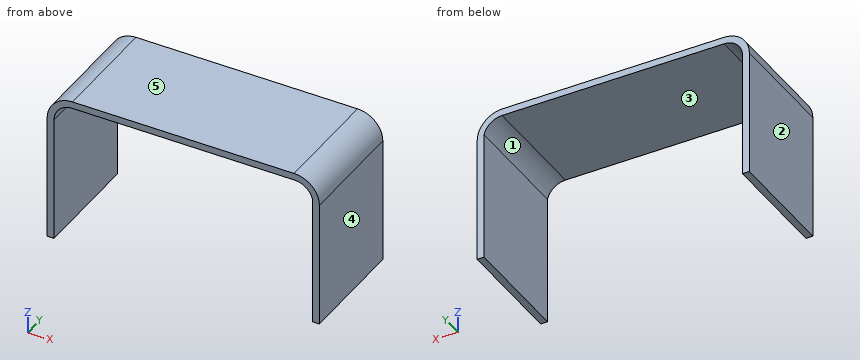
from build123d import *

# Parameters (mm, degrees)
F1_DEPTH = 147


with BuildPart() as f1:
    # F0 (on Front) → F1 (new body, symmetric)
    with BuildSketch(Plane.XZ):
        with BuildLine():
            Line((-1558.323113, 252.341221), (-1558.323113, -76.658779))
            Line((-1558.323113, -76.658779), (-1540.323113, -76.658779))
            Line((-1540.323113, -76.658779), (-1540.323113, 252.341221))
            ThreePointArc((-1540.323113, 252.341221), (-1526.264239, 286.282347), (-1492.323113, 300.341221))
            Line((-1492.323113, 300.341221), (-913.152471, 300.341221))
            ThreePointArc((-913.152471, 300.341221), (-883.16695, 289.822797), (-866.323113, 262.87741))
            Line((-866.323113, 262.87741), (-866.323113, -76.658779))
            Line((-866.323113, -76.658779), (-848.323113, -76.658779))
            Line((-848.323113, -76.658779), (-848.323113, 252.341221))
            ThreePointArc((-848.323113, 252.341221), (-867.654066, 299.010269), (-914.323113, 318.341221))
            Line((-914.323113, 318.341221), (-1492.323113, 318.341221))
            ThreePointArc((-1492.323113, 318.341221), (-1538.992161, 299.010269), (-1558.323113, 252.341221))
        make_face()
    extrude(amount=F1_DEPTH, both=True)


solid = f1.part
Verification items for the finished model (mm, model axes). Face numbers are marked on the shaded views. A direction names the side the tool comes from. Coordinates: 2 decimals unless noted, no trailing zeros. Loops run counter-clockwise (first coordinate to the right, second up) from the corner with the lowest first, then second, coordinate; pieces in that order, holes last. Notation, with made-up numbers: (-3, 63.25) -> (10, 63.25) arc R31 cw to (10, 99.25) -> close; hole circle Ø10 at (10, 56). An arc over 180 degrees is marked (long way). Answer as a JSON object with one key per item and string values. Group by question number.
Item 1: Sectioned sample at B-B on y = -24.5. Record the boundary of the cut face in (x, z), plus the area to 3 significant figures.
Item 2: Depth check by flat-ended pin: pin 1 (6 mm diameter, centred on x = -984, y = -61, fed in from -Z). Enter the tip coordinate at first touch or a pass-through.
Item 3: Sectioned sample at A-A on z = 241.5. Record the boundary of the cut face in (x, y), plus the area to 3 significant figures.
Item 4: Scan lines: probe 1 along X at (y, z) = (-63, 116.5); probe 2 along Z at (x, y) = (-996.5, -118); probe 3 along X at (y, z) = (-30, 274.5). Record each from-to range of solid material in increasing order.
Item 5: Tool access check on the marked faces 1 and 2. Record the directions out of +Z, -Z, +X, -X, +Y, -Y that give a thin tool (end or side, any length) a straight path to the whole face; none if there is none.
Item 6: Sectioned sample at C-C on x = -1265. Record the boundary of the cut face in (y, z).
Item 7: Mould release check, pull along X, two halves, no side actions. Record for the marked faces 3, 4 and 5: +X half, -X half, draft (parallel to the pull), parting line (faces both ways), or undercut.
Evaluation:
{
 "1": {"outline": "(-1558.32, -76.66) -> (-1540.32, -76.66) -> (-1540.32, 252.34) arc R48 cw to (-1492.32, 300.34) -> (-913.15, 300.34) arc R48 cw to (-866.32, 262.88) -> (-866.32, -76.66) -> (-848.32, -76.66) -> (-848.32, 252.34) arc R66 ccw to (-914.32, 318.34) -> (-1492.32, 318.34) arc R66 ccw to (-1558.32, 252.34) -> close", "area": "25,400 mm²"},
 "2": {"pin 1": "stops at z = 300.34"},
 "3": {"outline": "(-1558.32, -147) -> (-1540.32, -147) -> (-1540.32, 147) -> (-1558.32, 147) -> close; (-866.32, -147) -> (-848.32, -147) -> (-848.32, 147) -> (-866.32, 147) -> close", "area": "10,600 mm²"},
 "4": {"probe 1": "x = -1558.32 to -1540.32, -866.32 to -848.32", "probe 2": "z = 300.34 to 318.34", "probe 3": "x = -1554.49 to -1534.9, -870.57 to -852.15"},
 "5": {"face 1": "-Z, +Y, -Y", "face 2": "+Z, -Z, -X, +Y, -Y"},
 "6": {"outline": "(-147, 300.34) -> (147, 300.34) -> (147, 318.34) -> (-147, 318.34) -> close"},
 "7": {"face 3": "undercut", "face 4": "+X half", "face 5": "draft"}
}
